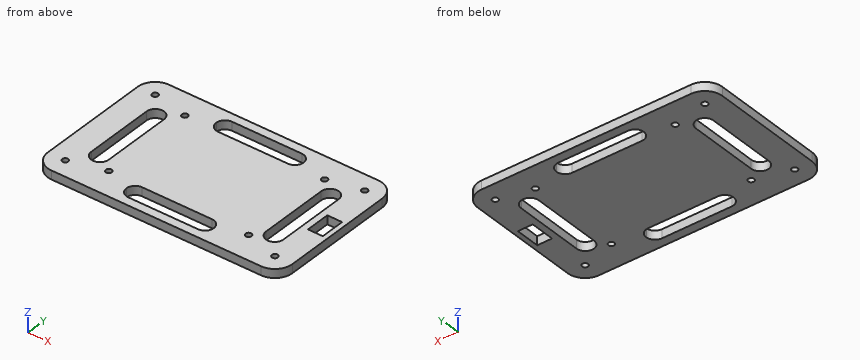
from build123d import *

# Parameters (mm, degrees)
BOSS_EXTRUDE1_DEPTH = 5
SKETCH2_R           = 1.7
SKETCH2_W           = 8.5
SKETCH2_H           = 14
CUT_EXTRUDE9_DEPTH  = 5


with BuildPart() as part:
    # Sketch1 → Boss-Extrude1 (new body)
    with BuildSketch(Plane.XY):
        with BuildLine():
            Line((-60, -42.5), (60, -42.5))
            ThreePointArc((60, -42.5), (67.071067812, -39.571067812), (70, -32.5))
            Line((70, -32.5), (70, 32.5))
            ThreePointArc((70, 32.5), (67.071067812, 39.571067812), (60, 42.5))
            Line((60, 42.5), (-60, 42.5))
            ThreePointArc((-60, 42.5), (-67.071067812, 39.571067812), (-70, 32.5))
            Line((-70, 32.5), (-70, -32.5))
            ThreePointArc((-70, -32.5), (-67.071067812, -39.571067812), (-60, -42.5))
        make_face()
    extrude(amount=BOSS_EXTRUDE1_DEPTH)

    # Sketch2 → Cut-Extrude9 (cut)
    with BuildSketch(Plane.XY):
        with BuildLine():
            Line((25, 32.5), (-25, 32.5))
            ThreePointArc((-25, 32.5), (-23.535533906, 28.964466094), (-20, 27.5))
            Line((-20, 27.5), (20, 27.5))
            ThreePointArc((20, 27.5), (23.535533906, 28.964466094), (25, 32.5))
        make_face()
        with BuildLine():
            ThreePointArc((-20, 37.5), (-23.535533906, 36.035533906), (-25, 32.5))
            Line((-25, 32.5), (25, 32.5))
            ThreePointArc((25, 32.5), (23.535533906, 36.035533906), (20, 37.5))
            Line((20, 37.5), (-20, 37.5))
        make_face()
        with BuildLine():
            Line((45, 20), (45, -20))
            ThreePointArc((45, -20), (50, -25), (55, -20))
            Line((55, -20), (55, 20))
            ThreePointArc((55, 20), (50, 25), (45, 20))
        make_face()
        with BuildLine():
            ThreePointArc((60, 34.2), (58.797918472, 31.297918472), (61.7, 32.5))
            Line((61.7, 32.5), (60, 32.5))
            Line((60, 32.5), (60, 34.2))
        make_face()
        with BuildLine():
            Line((60, 32.5), (61.7, 32.5))
            ThreePointArc((61.7, 32.5), (61.202081528, 33.702081528), (60, 34.2))
            Line((60, 34.2), (60, 32.5))
        make_face()
        with BuildLine():
            ThreePointArc((60, -34.2), (61.202081528, -33.702081528), (61.7, -32.5))
            Line((61.7, -32.5), (60, -32.5))
            Line((60, -32.5), (60, -34.2))
        make_face()
        with BuildLine():
            Line((60, -32.5), (61.7, -32.5))
            ThreePointArc((61.7, -32.5), (58.797918472, -31.297918472), (60, -34.2))
            Line((60, -34.2), (60, -32.5))
        make_face()
        with Locations((40.5, -26.9)):
            Circle(SKETCH2_R)
        with BuildLine():
            ThreePointArc((-20, -27.5), (-23.535533906, -28.964466094), (-25, -32.5))
            Line((-25, -32.5), (25, -32.5))
            ThreePointArc((25, -32.5), (23.535533906, -28.964466094), (20, -27.5))
            Line((20, -27.5), (-20, -27.5))
        make_face()
        with BuildLine():
            Line((25, -32.5), (-25, -32.5))
            ThreePointArc((-25, -32.5), (-23.535533906, -36.035533906), (-20, -37.5))
            Line((-20, -37.5), (20, -37.5))
            ThreePointArc((20, -37.5), (23.535533906, -36.035533906), (25, -32.5))
        make_face()
        with Locations((-39.5, -26.9)):
            Circle(SKETCH2_R)
        with BuildLine():
            ThreePointArc((-37.8, 28.1), (-38.297918472, 29.302081528), (-39.5, 29.8))
            Line((-39.5, 29.8), (-39.5, 28.1))
            Line((-39.5, 28.1), (-41.2, 28.1))
            ThreePointArc((-41.2, 28.1), (-39.5, 26.4), (-37.8, 28.1))
        make_face()
        with BuildLine():
            Line((-39.5, 28.1), (-39.5, 29.8))
            ThreePointArc((-39.5, 29.8), (-40.702081528, 29.302081528), (-41.2, 28.1))
            Line((-41.2, 28.1), (-39.5, 28.1))
        make_face()
        with BuildLine():
            Line((-55, 20), (-55, -20))
            ThreePointArc((-55, -20), (-50, -25), (-45, -20))
            Line((-45, -20), (-45, 20))
            ThreePointArc((-45, 20), (-50, 25), (-55, 20))
        make_face()
        with BuildLine():
            ThreePointArc((-60, 34.2), (-61.202081528, 33.702081528), (-61.7, 32.5))
            Line((-61.7, 32.5), (-60, 32.5))
            Line((-60, 32.5), (-60, 34.2))
        make_face()
        with BuildLine():
            Line((-60, 32.5), (-61.7, 32.5))
            ThreePointArc((-61.7, 32.5), (-60, 30.8), (-58.3, 32.5))
            ThreePointArc((-58.3, 32.5), (-58.797918472, 33.702081528), (-60, 34.2))
            Line((-60, 34.2), (-60, 32.5))
        make_face()
        with BuildLine():
            ThreePointArc((-58.3, -32.5), (-60, -30.8), (-61.7, -32.5))
            Line((-61.7, -32.5), (-60, -32.5))
            Line((-60, -32.5), (-60, -34.2))
            ThreePointArc((-60, -34.2), (-58.797918472, -33.702081528), (-58.3, -32.5))
        make_face()
        with BuildLine():
            Line((-60, -32.5), (-61.7, -32.5))
            ThreePointArc((-61.7, -32.5), (-61.202081528, -33.702081528), (-60, -34.2))
            Line((-60, -34.2), (-60, -32.5))
        make_face()
        with Locations((40.5, 28.1)):
            Circle(SKETCH2_R)
        with Locations((62.995775603, 0)):
            Rectangle(SKETCH2_W, SKETCH2_H)
    extrude(amount=CUT_EXTRUDE9_DEPTH, mode=Mode.SUBTRACT)


solid = part.part
Input: part model. Units: mm. Frame: model coordinates. Coordinates: 2 decimals unless noted, no trailing zeros. Loops run counter-clockwise (first coordinate to the right, second up) from the corner with the lowest first, then second, coordinate; pieces in that order, holes last.
(1) Section A-A on x = 15.5. Return the cut outline in (y, z), then the cut area to 3 significant figures.
(2) Material intervals for probe 1 along X at (y, z) = (32.5, 2.75); probe 2 along Y at (x, z) = (60, 3.8); probe 3 along Y at (x, z) = (40.5, 3.25), sorted ascending.
(3) Section B-B on y = -21.5. Return the cut outline in (x, z).
(4) Section C-C on z = 3.15. Count the separate pieces of the cut face and the enclosed holes in it, then the cut area to 3 significant figures.
Data:
1. outline: (-42.5, 0) - (-37.5, 0) - (-37.5, 5) - (-42.5, 5) - close; (-27.5, 0) - (27.5, 0) - (27.5, 5) - (-27.5, 5) - close; (37.5, 0) - (42.5, 0) - (42.5, 5) - (37.5, 5) - close
1. area: 325 mm2
2. probe 1: x = -70 to -61.7, -58.3 to -25, 25 to 58.3, 61.7 to 70
2. probe 2: y = -42.5 to -34.2, -30.8 to -7, 7 to 30.8, 34.2 to 42.5
2. probe 3: y = -42.5 to -28.6, -25.2 to 26.4, 29.8 to 42.5
3. outline: (-70, 0) - (-54.77, 0) - (-54.77, 5) - (-70, 5) - close; (-45.23, 0) - (45.23, 0) - (45.23, 5) - (-45.23, 5) - close; (54.77, 0) - (70, 0) - (70, 5) - (54.77, 5) - close
4. separate pieces: 1
4. enclosed holes: 13
4. area: 9,710 mm2
